```python
from build123d import *

# Parameters (mm, degrees)
SKETCH1_R           = 18.80108
BOSS_EXTRUDE1_DEPTH = 62
SKETCH2_R           = 1.58
BOSS_EXTRUDE2_DEPTH = 23
SKETCH3_R           = 1.5
CUT_EXTRUDE1_DEPTH  = 2
SKETCH4_R           = 6.5
BOSS_EXTRUDE3_DEPTH = 2


with BuildPart() as part:
    # Sketch1 → Boss-Extrude1 (new body)
    with BuildSketch(Plane(origin=(0, 0, 0), x_dir=(1, 0, 0), z_dir=(0, 1, 0))):
        with Locations(Location((0, 0, 0), (0, 0, 270))):
            Circle(SKETCH1_R)
    extrude(amount=-BOSS_EXTRUDE1_DEPTH)

    # Sketch2 → Boss-Extrude2 (add)
    with BuildSketch(Plane(origin=(0, 0, 0), x_dir=(1, 0, 0), z_dir=(0, 1, 0))):
        with Locations(Location((0, 0, 0), (0, 0, 270))):
            Circle(SKETCH2_R)
    extrude(amount=BOSS_EXTRUDE2_DEPTH)

    # Sketch3 → Cut-Extrude1 (cut)
    with BuildSketch(Plane(origin=(0, 0, 0), x_dir=(1, 0, 0), z_dir=(0, 1, 0))):
        with Locations(Location((0, 12.5, 0), (0, 0, 270))):
            Circle(SKETCH3_R)
        with Locations(Location((0, -12.5, 0), (0, 0, 270))):
            Circle(SKETCH3_R)
    extrude(amount=-CUT_EXTRUDE1_DEPTH, mode=Mode.SUBTRACT)

    # Sketch4 → Boss-Extrude3 (add)
    with BuildSketch(Plane(origin=(0, 0, 0), x_dir=(1, 0, 0), z_dir=(0, 1, 0))):
        with Locations(Location((0, 0, 0), (0, 0, 270))):
            Circle(SKETCH4_R)
    extrude(amount=BOSS_EXTRUDE3_DEPTH)


solid = part.part
```
CAD build for the part. Positions are in the model's coordinates, mm. A direction names the side the tool comes from. Give positions to 0.01 mm unless a question says otherwise; leave off trailing zeros. Order: outer loops, then holes, each group sorted by start corner. A loop starts at its lowest first (then second) coordinate and runs counter-clockwise, first axis right, second up.
(1) Flat gauge pins, fed straight in: pin 1 (1.8 mm diameter, centred on x = 0, z = 12.5, fed in from +Y); pin 2 (4 mm diameter, centred on x = -4.5, z = -10, fed in from +Y); pin 3 (2 mm diameter, centred on x = 7.5, y = -20.5, fed in from -Z). Where does each tip first touch, or does it go through?
(2) Saw through at B-B, the plane y = 9.5. Give the cut face in (x, z).
(3) Saw through at A-A, the plane z = 0. Give the cut face in (x, y), then the cut area to 3 significant figures.
(4) Drill centre lines: L1, parallel to Y at x = -10, z = 3; L2, parallel to X at y = -1.1, z = -12.5; L3, parallel to Y at x = 2.5, z = 0. Where is each one in solid material? Low to high.
(5) Saw through at C-C, the plane x = 15. Give the cut face in (y, z).
(6) Tool access for faces 1 (the cylindrical face through (1.567, 12.353, -0.206)), 2 (the flat face through (0, 23, 0)): list every direction of +Z, -Z, +X, -X, +Y, -Y with a clear straight run to the whole face (end or side of a thin tool).
(7) Saw through at D-D, the plane z = 4. Give the cut face in (x, y).
Results found:
1. pin 1: stops at y = -2
1. pin 2: stops at y = 0
1. pin 3: stops at z = -17.64
2. outline: circle Ø3.16 at (0, 0)
3. outline: (-18.8, -62) - (18.8, -62) - (18.8, 0) - (6.5, 0) - (6.5, 2) - (1.58, 2) - (1.58, 23) - (-1.58, 23) - (-1.58, 2) - (-6.5, 2) - (-6.5, 0) - (-18.8, 0) - close
3. area: 2,420 mm2
4. L1: y = -62 to 0
4. L2: x = -14.04 to -1.5, 1.5 to 14.04
4. L3: y = -62 to 2
5. outline: (-62, -11.33) - (0, -11.33) - (0, 11.33) - (-62, 11.33) - close
6. face 1: +Y
6. face 2: +Z, -Z, +X, -X, +Y
7. outline: (-18.37, -62) - (18.37, -62) - (18.37, 0) - (5.12, 0) - (5.12, 2) - (-5.12, 2) - (-5.12, 0) - (-18.37, 0) - close
